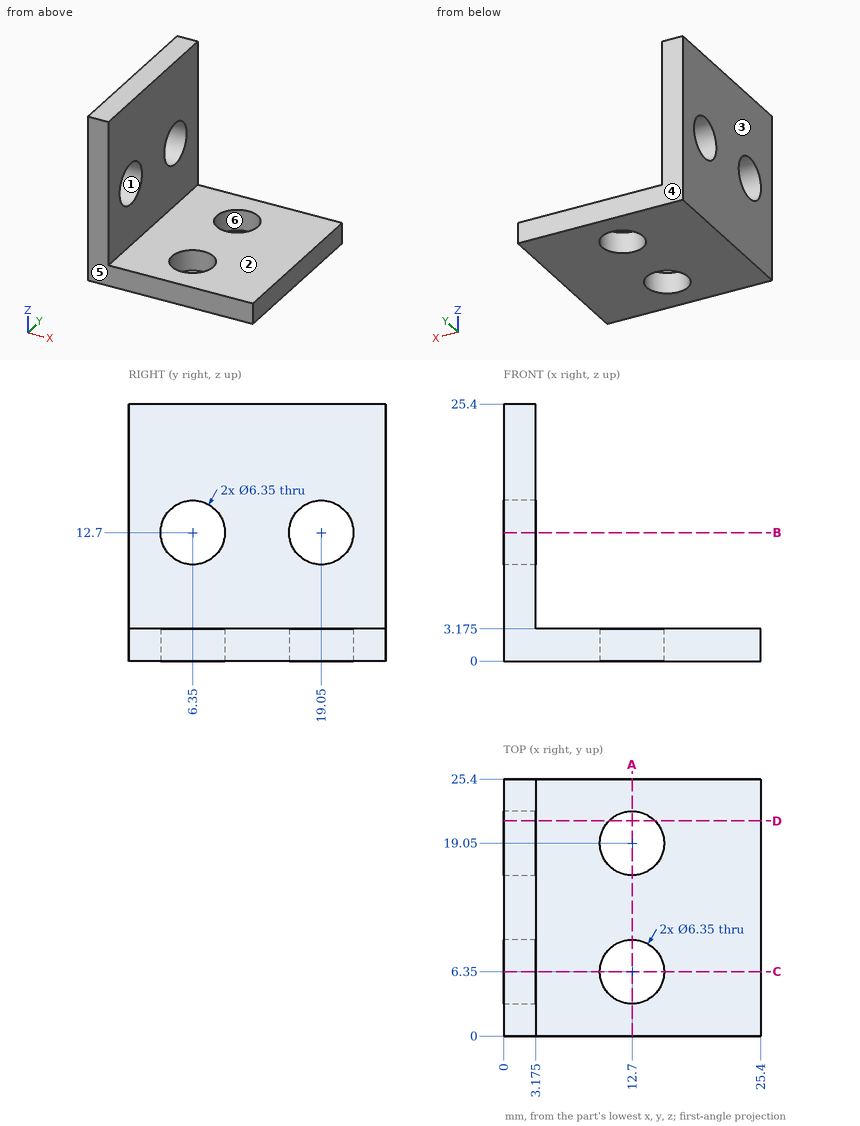
Source: three-view drawing plus pictorial views. Frame: mm from the lowest corner of the part. A direction names the side the tool comes from. Coordinates: 2 decimals unless noted, no trailing zeros. Write each loop counter-clockwise with the first axis right and the second up, starting at its lowest first coordinate (ties: lowest second). Pieces come first, ordered by that corner, then holes. Notation, with made-up numbers: (-10, 41.5) - (2, 41.5) arc R7 cw to (2, 53.5) - close; hole circle Ø4 at (-25, 42.25). An arc over 180 degrees is marked (long way). Answer as a JSON object with one key per item and string values.
Q1. Set-up query: the marked faces 1 and 2. Return all of +Z, -Z, +X, -X, +Y, -Y with unobstructed straight access to the full face (end or side cutting, diameter ignored); none if empty.
Ans:
{"face 1": "+X, -X", "face 2": "+Z, +X, +Y, -Y"}
Q2. Section query B-B, the plane z = 12.7. Output: boundary loops of the cut face in (x, y) (3 decimals), plus the area to 3 significant figures.
Ans:
{"outline": "(0, 0) - (3.175, 0) - (3.175, 3.175) - (0, 3.175) - close; (0, 9.525) - (3.175, 9.525) - (3.175, 15.875) - (0, 15.875) - close; (0, 22.225) - (3.175, 22.225) - (3.175, 25.4) - (0, 25.4) - close", "area": "40.3 mm2"}
Q3. Material intervals for line 1 (Z direction, x = 1.5, y = 19.05) (3 decimals); line 2 (X direction, y = 22, z = 5.5) (3 decimals), sorted ascending. Write a range as [from, to].
Ans:
{"line 1": "z = [0, 9.525], [15.875, 25.4]", "line 2": "x = [0, 3.175]"}
Q4. First-contact query: pin 1 Ø8.5 at (x, y) = (12.7, 6.35) entering from +Z (3 decimals); pin 2 Ø12 at (y, z) = (11.5, 17.5) entering from +X (3 decimals); pin 3 Ø8 at (x, y) = (19, 18.5) entering from -Z. Flat tips, straight axial feed; report the tip coordinate or a pass-through.
Ans:
{"pin 1": "stops at z = 3.175", "pin 2": "stops at x = 3.175", "pin 3": "stops at z = 0"}
Q5. Section query A-A, the plane x = 12.7. Output: boundary loops of the cut face in (y, z) (3 decimals).
Ans:
{"outline": "(0, 0) - (3.175, 0) - (3.175, 3.175) - (0, 3.175) - close; (9.525, 0) - (15.875, 0) - (15.875, 3.175) - (9.525, 3.175) - close; (22.225, 0) - (25.4, 0) - (25.4, 3.175) - (22.225, 3.175) - close"}
Q6. Section query D-D, the plane y = 21.25. Output: boundary loops of the cut face in (x, z) (3 decimals), plus the area to 3 significant figures.
Ans:
{"outline": "(0, 0) - (10.411, 0) - (10.411, 3.175) - (3.175, 3.175) - (3.175, 10.411) - (0, 10.411) - close; (0, 14.989) - (3.175, 14.989) - (3.175, 25.4) - (0, 25.4) - close; (14.989, 0) - (25.4, 0) - (25.4, 3.175) - (14.989, 3.175) - close", "area": "122 mm2"}
Q7. Draft query along Y for the marked faces 3, 4, 5 and 6. Return one class per face: released by +Y, released by -Y, zero draft, split by the parting line, or undercut.
Ans:
{"face 3": "zero draft", "face 4": "released by +Y", "face 5": "released by -Y", "face 6": "undercut"}
Q8. Section query C-C, the plane y = 6.35. Output: boundary loops of the cut face in (x, z) (3 decimals), plus the area to 3 significant figures.
Ans:
{"outline": "(0, 0) - (9.525, 0) - (9.525, 3.175) - (3.175, 3.175) - (3.175, 9.525) - (0, 9.525) - close; (0, 15.875) - (3.175, 15.875) - (3.175, 25.4) - (0, 25.4) - close; (15.875, 0) - (25.4, 0) - (25.4, 3.175) - (15.875, 3.175) - close", "area": "111 mm2"}
